```python
from build123d import *

# Parameters (mm, degrees)
SKETCH1_W           = 190
SKETCH1_H           = 195
BOSS_EXTRUDE1_DEPTH = 66.2
FILLET1_R           = 5
SKETCH2_R           = 1.7
CUT_EXTRUDE1_DEPTH  = 5
SKETCH3_R           = 7.5
BOSS_EXTRUDE2_DEPTH = 2
SKETCH4_W           = 15.7
SKETCH4_H           = 7.5
CUT_EXTRUDE2_DEPTH  = 5


with BuildPart() as part:
    # Sketch1 → Boss-Extrude1 (new body)
    with BuildSketch(Plane(origin=(0, 0, 0), x_dir=(1, 0, 0), z_dir=(0, 1, 0))):
        Rectangle(SKETCH1_W, SKETCH1_H)
    extrude(amount=BOSS_EXTRUDE1_DEPTH)

    # Fillet1
    fillet1_edges = [part.edges().sort_by_distance(p)[0] for p in [
        (-95, 66.2, 0),
        (95, 66.2, 0),
    ]]
    fillet(fillet1_edges, radius=FILLET1_R)

    # Sketch2 → Cut-Extrude1 (cut)
    with BuildSketch(Plane(origin=(0, 0, 0), x_dir=(-1, 0, 0), z_dir=(0, -1, 0))):
        with Locations(Location((85.725, -45, 0), (0, 0, 90))):
            Circle(SKETCH2_R)
        with Locations(Location((-85.725, -45, 0), (0, 0, 90))):
            Circle(SKETCH2_R)
        with Locations(Location((-85.725, 45, 0), (0, 0, 90))):
            Circle(SKETCH2_R)
        with Locations(Location((85.725, 45, 0), (0, 0, 90))):
            Circle(SKETCH2_R)
    extrude(amount=-CUT_EXTRUDE1_DEPTH, mode=Mode.SUBTRACT)

    # Sketch3 → Boss-Extrude2 (add)
    with BuildSketch(Plane.XY.offset(97.5)):
        with Locations(Location((-67, 45, 0), (0, 0, 180))):
            Circle(SKETCH3_R)
    extrude(amount=BOSS_EXTRUDE2_DEPTH)

    # Sketch4 → Cut-Extrude2 (cut)
    with BuildSketch(Plane.XY.offset(97.5)):
        with Locations((38, 51.2)):
            Rectangle(SKETCH4_W, SKETCH4_H)
        with Locations((60, 51.2)):
            Rectangle(SKETCH4_W, SKETCH4_H)
    extrude(amount=-CUT_EXTRUDE2_DEPTH, mode=Mode.SUBTRACT)


solid = part.part
```
Work out the finished part from the listing and answer in its coordinate system (mm). A direction names the side the tool comes from. Round coordinates to 2 decimals unless told otherwise and drop trailing zeros.
(1) For faces 4 (the flat face through (-67, 45, 99.5)), 5 (the flat face through (45.85, 51, 95)), determine the directions among +Z, -Z, +X, -X, +Y, -Y from which every point of the face is accessible in a straight line to the end or side of a thin tool.
Computed values:
face 4: +Z, +X, -X, +Y, -Y
face 5: +Z
(2) The mould has two halves that part along Y. Classify faces 1 (the cylindrical face through (93.57, 64.7, -1.36)), 2 (the flat face through (60, 47.45, 95)), 3 (the flat face through (95, 30, 1)): pulls with the +Y half, pulls with the -Y half, needs draft (parallel to the pull), parting line crosses it, or undercut.
Computed values:
face 1: pulls with the +Y half
face 2: undercut
face 3: needs draft
(3) Find the intervals of material crossed by L1, parallel to X at y = 2.85, z = 45 (3 decimals); L2, parallel to Z at x = 27, y = 18, in increasing order.
Computed values:
L1: x = -95 to -87.425, -84.025 to 84.025, 87.425 to 95
L2: z = -97.5 to 97.5
(4) Each of these flat-tipped pins is pushed along its axis until it touches: P1, Ø4, axis at x = 37.5, z = 94, coming from the -Y side; P2, Ø4, axis at x = 59.5, y = 50, coming from the +Z side. Where does it stop, or does it pass through?
Computed values:
P1: stops at y = 0
P2: stops at z = 92.5
